Build history of the part. All positions in model axes, mm. A direction names the side the tool comes from. Round coordinates to 2 decimals unless told otherwise and drop trailing zeros. Write each loop counter-clockwise with the first axis right and the second up, starting at its lowest first coordinate (ties: lowest second). Pieces come first, ordered by that corner, then holes.
Item 1: Band-saw the part on B-B, the plane z = 1. Write the cut outline in (x, y).
Item 2: Band-saw the part on A-A, the plane x = 92.5. Write the cut outline in (y, z).
Item 3: 3-axis set-ups, long thin cutter, end or side, ignore diameter. For faces 4 (the cylindrical face through (53.608, 22.062, -4.399)), 5 (the cylindrical face through (122.409, 47.276, 0.059)), 6 (the cylindrical face through (34.828, -12.684, -4.399)): which of +Z, -Z, +X, -X, +Y, -Y reach the whole face in a straight line?
Item 4: Band-saw the part on C-C, the plane x = 40. Count the separate pieces of the cut face and the enclosed holes in it, then the cut area to 3 significant figures.
Item 5: Drop flat-ended pins along their axis: pin 1 Ø1.8 at (x, z) = (95.5, -0.5) entering from -Y; pin 2 Ø2 at (y, z) = (21.5, -1) entering from +X; pin 3 Ø3 at (x, z) = (28, -1) entering from -Y; pin 4 Ø2 at (y, z) = (48, 0.5) entering from +X. Give the stop position or say it passes through.
Item 6: Mould opens along Z. For faces 1 (the flat face through (39.982, -10.266, 0.042)), 2 (the cylindrical face through (39.8, -9.5, -4.4)), 3 (the flat face through (118.86, 49, 0)) say: +Z half, -Z half, draft (parallel to the pull), parting line (faces both ways), or undercut.
Item 7: Wall check: probe 1 along Y at (x, z) = (32.5, -4.5); probe 2 along Y at (x, z) = (37, 1.25); probe 3 along Y at (x, z) = (95.5, 1.5). Give the ranges that are in metal, low to high.
```python
from build123d import *

# Parameters (mm, degrees)
BOSS_EXTRUDE1_DEPTH = 5
FILLET1_R           = 2
SKETCH2_R           = 3.125
CUT_EXTRUDE1_DEPTH  = 7
FILLET2_R           = 0.3


with BuildPart() as part:
    # Sketch1 → Boss-Extrude1 (new, symmetric)
    with BuildSketch(Plane.XY):
        Polygon((0, 0), (80.860254038, 50), (125.860254038, 50), (125.860254038, 40), (83.702282943, 40), (27.312387914, 5.13126523), (52.351270189, -9.324940192), (48.851270189, -15.387118018), (30.860254038, -5), (22.660254038, -5), (46.801270189, -18.937822174), (43.301270189, -25), align=None)
    extrude(amount=BOSS_EXTRUDE1_DEPTH, both=True)

    # Fillet1
    fillet1_edges = [part.edges().sort_by_distance(p)[0] for p in [
        (40.430127019, 25, -5),
        (103.360254038, 50, -5),
        (34.730762114, -11.968911087, 5),
        (125.860254038, 45, -5),
        (104.78126849, 40, -5),
        (55.507335428, 22.565632615, -5),
        (39.831829052, -2.096837481, -5),
        (50.601270189, -12.356029105, -5),
        (39.855762114, -10.193559009, -5),
        (26.760254038, -5, -5),
        (34.730762114, -11.968911087, -5),
        (45.051270189, -21.968911087, -5),
        (21.650635095, -12.5, -5),
        (26.760254038, -5, 5),
        (39.855762114, -10.193559009, 5),
        (50.601270189, -12.356029105, 5),
        (39.831829052, -2.096837481, 5),
        (55.507335428, 22.565632615, 5),
        (104.78126849, 40, 5),
        (125.860254038, 45, 5),
        (103.360254038, 50, 5),
        (40.430127019, 25, 5),
        (21.650635095, -12.5, 5),
        (45.051270189, -21.968911087, 5),
    ]]
    fillet(fillet1_edges, radius=FILLET1_R)

    # Sketch2 → Cut-Extrude1 (cut)
    with BuildSketch(Plane(origin=(125.860254038, 0, 0), x_dir=(0, 0, -1), z_dir=(1, 0, 0))):
        with Locations((0, 50.4)):
            Circle(SKETCH2_R)
    extrude(amount=-CUT_EXTRUDE1_DEPTH, mode=Mode.SUBTRACT)

    # Fillet2
    fillet2_edges = [part.edges().sort_by_distance(p)[0] for p in [
        (122.359028731, 49.997549387, 3.098977009),
        (122.359028731, 49.997549387, -3.098977009),
    ]]
    fillet(fillet2_edges, radius=FILLET2_R)


solid = part.part
```
Results:
1. outline: (0, 0) - (43.3, -25) - (46.8, -18.94) - (22.66, -5) - (30.86, -5) - (48.85, -15.39) - (52.35, -9.32) - (27.31, 5.13) - (83.7, 40) - (125.86, 40) - (125.86, 47.44) - (118.86, 47.44) - (118.86, 50) - (80.86, 50) - close
2. outline: (40, -3) arc R2 ccw to (42, -5) - (48, -5) arc R2 ccw to (50, -3) - (50, 3) arc R2 ccw to (48, 5) - (42, 5) arc R2 ccw to (40, 3) - close
3. face 4: -Z, +X
3. face 5: +X, +Y
3. face 6: -Z
4. separate pieces: 3
4. enclosed holes: 0
4. area: 267 mm2
5. pin 1: stops at y = 40
5. pin 2: stops at x = 55.4
5. pin 3: stops at y = -17.03
5. pin 4: stops at x = 125.86
6. face 1: draft
6. face 2: -Z half
6. face 3: undercut
7. probe 1: y = -17.98 to -11.46, -5.16 to 1.35, 9.14 to 19.3
7. probe 2: y = -21.36 to -13.28, -8.54 to -0.46, 11.12 to 22.88
7. probe 3: y = 40 to 50
